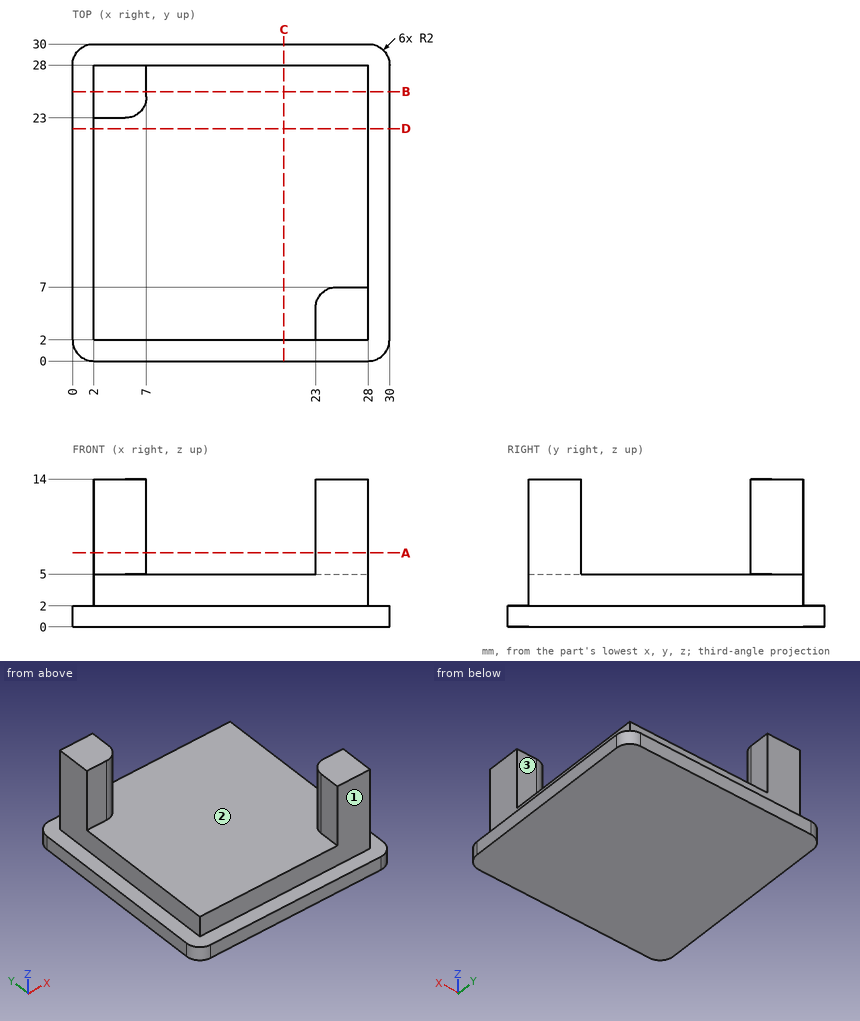
Design review of the part shown in the three views and the two pictorial views. Dimensions are in mm from the part's minimum x, y and z. A direction names the side the tool comes from. Round coordinates to 2 decimals unless told otherwise and drop trailing zeros. Loops run counter-clockwise (first coordinate to the right, second up) from the corner with the lowest first, then second, coordinate; pieces in that order, holes last. Notation, with made-up numbers: (47, -36) -> (85, -36) arc R16 cw to (85, -7) -> close; hole circle Ø11 at (33, -1). An arc over 180 degrees is marked (long way). Answer as a JSON object with one key per item and string values. Group by question number.
1) We need section C-C on x = 20. Write out the cut boundary in (y, z).
2) We need section B-B on y = 25.5. Write out the cut boundary in (x, z).
3) We need section A-A on z = 7. Write out the cut boundary in (x, y), then the cut area to 3 significant figures.
4) For pin 1 Ø3.5 at (y, z) = (11.5, 6) entering from -X; pin 2 Ø8 at (y, z) = (3.5, 10) entering from -X; pin 3 Ø6 at (x, y) = (6.5, 16.5) entering from +Z, all flat-tipped, find the tip position at first contact; note any pin that passes through.
5) For line 1 (Z direction, x = 9.75, y = 15.5); line 2 (Y direction, x = 3, z = 6.5); line 3 (Y direction, x = 6, z = 3), list the stretches that pass through material, from the lowest coordinate up. Write a range as [from, to].
6) For the marked faces 1, 2 and 3, list the 3-axis set-ups (+Z, -Z, +X, -X, +Y, -Y) from which the entire face can be reached by the end or side of a thin tool; tool diameter is ignored.
Result set:
{
 "1": {"outline": "(0, 0) -> (30, 0) -> (30, 2) -> (28, 2) -> (28, 5) -> (2, 5) -> (2, 2) -> (0, 2) -> close"},
 "2": {"outline": "(0, 0) -> (30, 0) -> (30, 2) -> (28, 2) -> (28, 5) -> (7, 5) -> (7, 14) -> (2, 14) -> (2, 2) -> (0, 2) -> close"},
 "3": {"outline": "(2, 23) -> (5, 23) arc R2 ccw to (7, 25) -> (7, 28) -> (2, 28) -> close; (23, 2) -> (28, 2) -> (28, 7) -> (25, 7) arc R2 ccw to (23, 5) -> close", "area": "48.3 mm²"},
 "4": {"pin 1": "x = 2", "pin 2": "x = 23", "pin 3": "z = 5"},
 "5": {"line 1": "[0, 5]", "line 2": "[23, 28]", "line 3": "[2, 28]"},
 "6": {"face 1": "+Z, +X, -X, -Y", "face 2": "+Z", "face 3": "+Z, +X, -X, +Y"}
}
